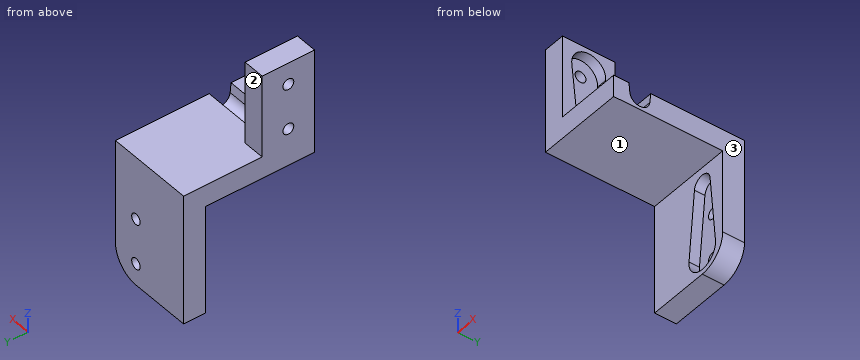
```python
from build123d import *

# Parameters (mm, degrees)
SKETCH1_W               = 20
SKETCH1_H               = 30
BOSS_EXTRUDE1_DEPTH     = 5
CUT_EXTRUDE1_DEPTH      = 2.4
SKETCH7_R               = 1.25
CUT_EXTRUDE4_DEPTH      = 19.214280112
BOSS_EXTRUDE2_DEPTH     = 10
SKETCH5_W               = 19
SKETCH5_H               = 12
CUT_EXTRUDE2_DEPTH      = 15
CUT_EXTRUDE3_DEPTH      = 45.788391353
CUT_EXTRUDE3_DEPTH_BACK = 2.4
SKETCH8_R               = 1.25
CUT_EXTRUDE5_DEPTH      = 46.648220119
FILLET1_R               = 6


with BuildPart() as part:
    # Sketch1 → Boss-Extrude1 (new body)
    with BuildSketch(Plane(origin=(0, 0, 0), x_dir=(1, 0, 0), z_dir=(0, 1, 0))):
        Rectangle(SKETCH1_W, SKETCH1_H)
    extrude(amount=BOSS_EXTRUDE1_DEPTH)

    # Sketch2 → Cut-Extrude1 (cut)
    with BuildSketch(Plane.XZ):
        with BuildLine():
            Line((0.119672063, -9.608777429), (1.711601473, 6.180721003))
            ThreePointArc((1.711601473, 6.180721003), (4, 8.25), (6.288398527, 6.180721003))
            Line((6.288398527, 6.180721003), (7.880327937, -9.608777429))
            ThreePointArc((7.880327937, -9.608777429), (4, -13.9), (0.119672063, -9.608777429))
        make_face()
    extrude(amount=-CUT_EXTRUDE1_DEPTH, mode=Mode.SUBTRACT)

    # Sketch7 → Cut-Extrude4 (cut, through all)
    with BuildSketch(Plane.XZ.offset(-2.4)):
        with Locations(Location((4, -10, 0), (0, 0, 270))):
            Circle(SKETCH7_R)
        with Locations(Location((4, 0.45, 0), (0, 0, 270))):
            Circle(SKETCH7_R)
    extrude(amount=-CUT_EXTRUDE4_DEPTH, mode=Mode.SUBTRACT)

    # Sketch4 → Boss-Extrude2 (add, symmetric)
    with BuildSketch(Plane(origin=(0, 0, 0), x_dir=(0, 0, -1), z_dir=(1, 0, 0))):
        Polygon((-15, 0), (-10, 0), (-10, -25), (-15, -25), (-34, -25), (-34, -13), (-15, -13), align=None)
    extrude(amount=BOSS_EXTRUDE2_DEPTH, both=True)

    # Sketch5 → Cut-Extrude2 (cut)
    with BuildSketch(Plane(origin=(10, 0, 0), x_dir=(0, 0, -1), z_dir=(1, 0, 0))):
        with Locations((-24.5, -19)):
            Rectangle(SKETCH5_W, SKETCH5_H)
    extrude(amount=-CUT_EXTRUDE2_DEPTH, mode=Mode.SUBTRACT)

    # Sketch6 → Cut-Extrude3 (cut, two sides: drawn at the far end of the back side and taken through both)
    with BuildSketch(Plane(origin=(-5, 0, 0), x_dir=(0, 0, -1), z_dir=(1, 0, 0)).offset(-CUT_EXTRUDE3_DEPTH_BACK)):
        with BuildLine():
            Line((-28.608777429, -22.880327937), (-12.819278997, -21.288398527))
            ThreePointArc((-12.819278997, -21.288398527), (-10.75, -19), (-12.819278997, -16.711601473))
            Line((-12.819278997, -16.711601473), (-28.608777429, -15.119672063))
            ThreePointArc((-28.608777429, -15.119672063), (-32.9, -19), (-28.608777429, -22.880327937))
        make_face()
    extrude(amount=CUT_EXTRUDE3_DEPTH + CUT_EXTRUDE3_DEPTH_BACK, mode=Mode.SUBTRACT)

    # Sketch8 → Cut-Extrude5 (cut, through all)
    with BuildSketch(Plane(origin=(-7.4, 0, 0), x_dir=(0, 0, -1), z_dir=(1, 0, 0))):
        with Locations((-29, -19)):
            Circle(SKETCH8_R)
        with Locations((-18.55, -19)):
            Circle(SKETCH8_R)
    extrude(amount=-CUT_EXTRUDE5_DEPTH, mode=Mode.SUBTRACT)

    # Fillet1
    fillet1_edges = [part.edges().sort_by_distance(p)[0] for p in [
        (10, 2.5, -15),
    ]]
    fillet(fillet1_edges, radius=FILLET1_R)


solid = part.part
```
Model file for the job. Use its own axes, mm. Face numbers are marked on the shaded views. A direction names the side the tool comes from. Give positions to 0.01 mm unless a question says otherwise; leave off trailing zeros. Write each loop counter-clockwise with the first axis right and the second up, starting at its lowest first coordinate (ties: lowest second). Pieces come first, ordered by that corner, then holes. Notation, with made-up numbers: M -25.75,-6 L -11.75,-6 A21 ccw -11.75,0 Z; hole C 16.5,-33.75 d3. An arc over 180 degrees is marked long. Use a Markdown table: item, result.
1) Tool access for the marked faces 1, 2 and 3: list every direction of +Z, -Z, +X, -X, +Y, -Y with a clear straight run to the whole face (end or side of a thin tool).
Responses:
| item | result |
|---|---|
| face 1 | -Z, +X, -X, -Y |
| face 2 | +Z, +X, -X, +Y |
| face 3 | +Z, -Z, +X, +Y, -Y |
2) Drill centre lines: line 1 (Y direction, x = -6.45, z = 29); line 2 (Z direction, x = 3.75, y = -15); line 3 (Y direction, x = 1.5, z = -8). Where is each one in solid material? Low to high. Write a range as from..to.
Responses:
| item | result |
|---|---|
| line 1 | y = -25..-22.9, -15.1..-13 |
| line 2 | z = 10..15 |
| line 3 | y = 2.4..5 |
3) Cut at C-C (z = 18.55). List the corners of the cut face in (x, y), and give its area (3 significant figures).
Responses:
| item | result |
|---|---|
| outline | M -10,-25 L -5,-25 L -5,-21.87 L -7.4,-21.87 L -7.4,-20.25 L -10,-20.25 Z; M -10,-17.75 L -7.4,-17.75 L -7.4,-16.13 L -5,-16.13 L -5,-13 L -10,-13 Z |
| area | 39.7 mm2 |
4) Pin check, flat tips, straight feed: pin 1 (7 mm diameter, centred on y = -19, z = 29, fed in from +X); pin 2 (6 mm diameter, centred on x = 3.5, z = -0.5, fed in from -Y); pin 3 (3 mm diameter, centred on x = -5, y = -14.5, fed in from -Z). Stop position of each tip, or through.
Responses:
| item | result |
|---|---|
| pin 1 | stops at x = -7.4 |
| pin 2 | stops at y = 0 |
| pin 3 | stops at z = 10 |
5) Cut at A-A (x = -6). List the corners of the cut face in (y, z), and give its area (3 significant figures).
Responses:
| item | result |
|---|---|
| outline | M -25,10 L 0,10 L 0,-15 L 5,-15 L 5,15 L -13,15 L -13,34 L -25,34 Z; hole M -22.88,28.61 L -21.29,12.82 A2.3 ccw -16.71,12.82 L -15.12,28.61 A3.9 ccw long Z |
| area | 371 mm2 |
6) Cut at D-D (y = 0.5). List the corners of the cut face in (x, z).
Responses:
| item | result |
|---|---|
| outline | M -10,-15 L 4,-15 A6 ccw 10,-9 L 10,15 L -10,15 Z; hole M 0.12,-9.61 A3.9 ccw long 7.88,-9.61 L 6.29,6.18 A2.3 ccw 1.71,6.18 Z |
7) Cut at B-B (y = -19). List the corners of the cut face in (x, z), and give its area (3 significant figures).
Responses:
| item | result |
|---|---|
| outline | M -10,10 L 10,10 L 10,10.75 L -7.4,10.75 L -7.4,17.3 L -10,17.3 Z; M -10,19.8 L -7.4,19.8 L -7.4,27.75 L -10,27.75 Z; M -10,30.25 L -7.4,30.25 L -7.4,32.9 L -5,32.9 L -5,34 L -10,34 Z |
| area | 65.1 mm2 |
